Geometry: final body of the model. Coordinates: model frame, mm. A direction names the side the tool comes from. Give positions to 0.01 mm unless a question says otherwise; leave off trailing zeros. Write each loop counter-clockwise with the first axis right and the second up, starting at its lowest first coordinate (ties: lowest second). Pieces come first, ordered by that corner, then holes.
```python
from build123d import *

# Parameters (mm, degrees)
SKETCH1_W           = 76.2
SKETCH1_H           = 25.4
SKETCH1_W_2         = 69.85
SKETCH1_H_2         = 19.05
EXTRUDE_THIN1_DEPTH = 420.69258
SKETCH4_R           = 24.97201
CUT_EXTRUDE3_DEPTH  = 26.4
CUT_EXTRUDE7_DEPTH  = 26.4
SKETCH7_R           = 3.175
CUT_EXTRUDE8_DEPTH  = 77.2
SKETCH8_R           = 3.175
CUT_EXTRUDE9_DEPTH  = 77.2


with BuildPart() as part:
    # Sketch1 → Extrude-Thin1 (new body)
    with BuildSketch(Plane.XY):
        Rectangle(SKETCH1_W, SKETCH1_H)
        Rectangle(SKETCH1_W_2, SKETCH1_H_2, mode=Mode.SUBTRACT)
    extrude(amount=EXTRUDE_THIN1_DEPTH)

    # Sketch4 → Cut-Extrude3 (cut, through all)
    with BuildSketch(Plane(origin=(0, 12.7, 0), x_dir=(1, 0, 0), z_dir=(0, 1, 0))):
        with Locations((0, -361.82808)):
            Circle(SKETCH4_R)
        with Locations((0, -58.8645)):
            Circle(SKETCH4_R)
    extrude(amount=-CUT_EXTRUDE3_DEPTH, mode=Mode.SUBTRACT)

    # Sketch6 → Cut-Extrude7 (cut, through all)
    with BuildSketch(Plane(origin=(0, 12.7, 0), x_dir=(1, 0, 0), z_dir=(0, 1, 0))):
        with BuildLine():
            Line((23.8125, 0), (-25.4, 0))
            Line((-25.4, 0), (-25.4, -32.480924163))
            ThreePointArc((-25.4, -32.480924163), (-23.564047105, -35.359739519), (-20.179478519, -34.909188331))
            ThreePointArc((-20.179478519, -34.909188331), (-0.919958513, -27.556002962), (18.738087196, -33.765647463))
            ThreePointArc((18.738087196, -33.765647463), (22.060523075, -34.059710885), (23.8125, -31.221466652))
            Line((23.8125, -31.221466652), (23.8125, 0))
        make_face()
    cut_extrude7 = extrude(amount=-CUT_EXTRUDE7_DEPTH, mode=Mode.SUBTRACT)

    # Sketch7 → Cut-Extrude8 (cut, through all)
    with BuildSketch(Plane(origin=(38.1, 0, 0), x_dir=(0, 0, -1), z_dir=(1, 0, 0))):
        with Locations((-14.4145, 0)):
            Circle(SKETCH7_R)
    cut_extrude8 = extrude(amount=-CUT_EXTRUDE8_DEPTH, mode=Mode.SUBTRACT)

    # Mirror3: Cut-Extrude7, Cut-Extrude8 across plane
    add(cut_extrude7.mirror(Plane.XY.offset(210.34629)), mode=Mode.SUBTRACT)
    add(cut_extrude8.mirror(Plane.XY.offset(210.34629)), mode=Mode.SUBTRACT)

    # Sketch8 → Cut-Extrude9 (cut, through all)
    with BuildSketch(Plane(origin=(38.1, 0, 0), x_dir=(0, 0, -1), z_dir=(1, 0, 0))):
        with Locations((-58.8645, 0)):
            Circle(SKETCH8_R)
        with Locations((-361.82808, 0)):
            Circle(SKETCH8_R)
    extrude(amount=-CUT_EXTRUDE9_DEPTH, mode=Mode.SUBTRACT)


solid = part.part
```
Item 1: Reachability of faces 1 (the face through (-36, 0, 0)), 2 (the face through (-34.925, 0, 207)) from +Z, -Z, +X, -X, +Y, -Y: full face, straight path, thin tool, end or side. Return the list, or none.
Found:
face 1: -Z, +X, -X, +Y, -Y
face 2: +Z, -Z
Item 2: Line query: L1, parallel to Z at x = 0, y = -11; L2, parallel to Y at x = 28, z = 225 (3 decimals); L3, parallel to X at y = -1, z = 168.5 (3 decimals). Output: solid intervals per line, ascending.
Found:
L1: z = 27.54 to 33.89, 83.84 to 336.86, 386.8 to 393.15
L2: y = -12.7 to -9.525, 9.525 to 12.7
L3: x = -38.1 to -34.925, 34.925 to 38.1
Item 3: Section C-C, the plane x = 15. Return the cut outline in (y, z) (1 decimal).
Found:
outline: (-12.7, 31.4) - (-9.5, 31.4) - (-9.5, 38.9) - (-12.7, 38.9) - close; (-12.7, 78.8) - (-9.5, 78.8) - (-9.5, 341.9) - (-12.7, 341.9) - close; (-12.7, 381.8) - (-9.5, 381.8) - (-9.5, 389.3) - (-12.7, 389.3) - close; (9.5, 31.4) - (12.7, 31.4) - (12.7, 38.9) - (9.5, 38.9) - close; (9.5, 78.8) - (12.7, 78.8) - (12.7, 341.9) - (9.5, 341.9) - close; (9.5, 381.8) - (12.7, 381.8) - (12.7, 389.3) - (9.5, 389.3) - close
Item 4: Section B-B, the plane x = 0. Return the cut outline in (y, z) (3 decimals), plus the area to 3 significant figures.
Found:
outline: (-12.7, 27.542) - (-9.525, 27.542) - (-9.525, 33.892) - (-12.7, 33.892) - close; (-12.7, 83.837) - (-9.525, 83.837) - (-9.525, 336.856) - (-12.7, 336.856) - close; (-12.7, 386.8) - (-9.525, 386.8) - (-9.525, 393.15) - (-12.7, 393.15) - close; (9.525, 27.542) - (12.7, 27.542) - (12.7, 33.892) - (9.525, 33.892) - close; (9.525, 83.837) - (12.7, 83.837) - (12.7, 336.856) - (9.525, 336.856) - close; (9.525, 386.8) - (12.7, 386.8) - (12.7, 393.15) - (9.525, 393.15) - close
area: 1,690 mm2
Item 5: Pull-direction query (Y, two-part tool) for faces 3 (the face through (-1, -12.7, 207)), 4 (the face through (34.925, 0, 207)), 5 (the face through (0, 9.525, 207)), 6 (the face through (-5.413, 11.135, 386.206)); classes: +Y half, -Y half, draft (parallel to the pull), parting line (faces both ways), or undercut.
Found:
face 3: -Y half
face 4: undercut
face 5: undercut
face 6: draft
Item 6: Section A-A, the plane z = 305.5. Return the cut outline in (x, y) (3 decimals).
Found:
outline: (-38.1, -12.7) - (38.1, -12.7) - (38.1, 12.7) - (-38.1, 12.7) - close; hole (-34.925, -9.525) - (34.925, -9.525) - (34.925, 9.525) - (-34.925, 9.525) - close
Item 7: Pin query (flat end, axial travel): pin 1 Ø10 at (y, z) = (0, 361.83) entering from +X. Return the tip coordinate at first contact, or that it passes through.
Found:
pin 1: stops at x = 38.1
